Input: part model. Units: mm. Frame: model coordinates. Round coordinates to 2 decimals unless told otherwise and drop trailing zeros. Loops run counter-clockwise (first coordinate to the right, second up) from the corner with the lowest first, then second, coordinate; pieces in that order, holes last. Notation, with made-up numbers: (19, 23.5) -> (35, 23.5) arc R20 cw to (35, 28.5) -> close; hole circle Ø9 at (67, 50.5). An arc over 180 degrees is marked (long way). Answer as a JSON object with one key per item and string values.
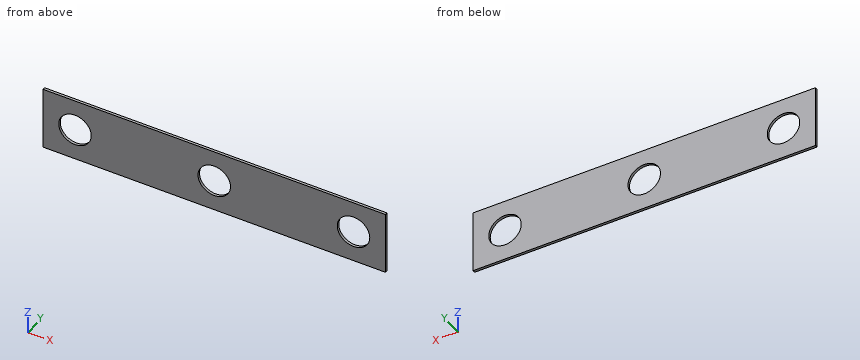
```python
from build123d import *

# Parameters (mm, degrees)
SKETCH1_W                 = 17
SKETCH1_H                 = 3.175
BOSS_EXTRUDE1_DEPTH       = 0.127
F_0_CLEARANCE_HOLE1_D     = 1.6129
F_0_CLEARANCE_HOLE1_DEPTH = 4.826
F_0_CLEARANCE_HOLE1_TIP   = 0.484564046


with BuildPart() as part:
    # Sketch1 → Boss-Extrude1 (new body)
    with BuildSketch(Plane(origin=(0, 0, 0), x_dir=(1, 0, 0), z_dir=(0, 1, 0))):
        Rectangle(SKETCH1_W, SKETCH1_H)
    extrude(amount=BOSS_EXTRUDE1_DEPTH)

    # #0 Clearance Hole1
    with Locations(Plane(origin=(0, 0.127, 0), x_dir=(-1, 0, 0), z_dir=(0, 1, 0))):
        with Locations((0, 0), (-6.9125, 0), (6.9125, 0)):
            Hole(F_0_CLEARANCE_HOLE1_D / 2, depth=F_0_CLEARANCE_HOLE1_DEPTH)
            with Locations((0, 0, -(F_0_CLEARANCE_HOLE1_DEPTH + F_0_CLEARANCE_HOLE1_TIP / 2))):  # 118° drill point
                Cone(0, F_0_CLEARANCE_HOLE1_D / 2, F_0_CLEARANCE_HOLE1_TIP, mode=Mode.SUBTRACT)


solid = part.part
```
1) Section B-B, the plane z = 0. Output: boundary loops of the cut face in (x, y), plus the area to 3 significant figures.
Output:
{"outline": "(-8.5, 0) -> (-7.72, 0) -> (-7.72, 0.13) -> (-8.5, 0.13) -> close; (-6.11, 0) -> (-0.81, 0) -> (-0.81, 0.13) -> (-6.11, 0.13) -> close; (0.81, 0) -> (6.11, 0) -> (6.11, 0.13) -> (0.81, 0.13) -> close; (7.72, 0) -> (8.5, 0) -> (8.5, 0.13) -> (7.72, 0.13) -> close", "area": "1.54 mm^2"}
2) Section A-A, the plane x = 0. Output: boundary loops of the cut face in (y, z).
Output:
{"outline": "(0, -1.59) -> (0.13, -1.59) -> (0.13, -0.81) -> (0, -0.81) -> close; (0, 0.81) -> (0.13, 0.81) -> (0.13, 1.59) -> (0, 1.59) -> close"}
3) Ray query, probe 1 along X at (y, z) = (0.05, -0.4); probe 2 along Z at (x, y) = (0, 0.05). Return the intervals inside material, ascending.
Output:
{"probe 1": "x = -8.5 to -7.61, -6.21 to -0.7, 0.7 to 6.21, 7.61 to 8.5", "probe 2": "z = -1.59 to -0.81, 0.81 to 1.59"}
